Study the drawing (mm; zero at the part's minimum x, y, z) and answer. A direction names the side the tool comes from. Round coordinates to 2 decimals unless told otherwise and drop trailing zeros. Order: outer loops, then holes, each group sorted by start corner. A loop starts at its lowest first (then second) coordinate and runs counter-clockwise, first axis right, second up. Notation, with made-up numbers: (58, 4.5) - (86, 4.5) arc R17 cw to (86, 29.5) - close; hole circle Ø7 at (70, 44). An arc over 180 degrees is marked (long way). Put each result on its own line as item: value.
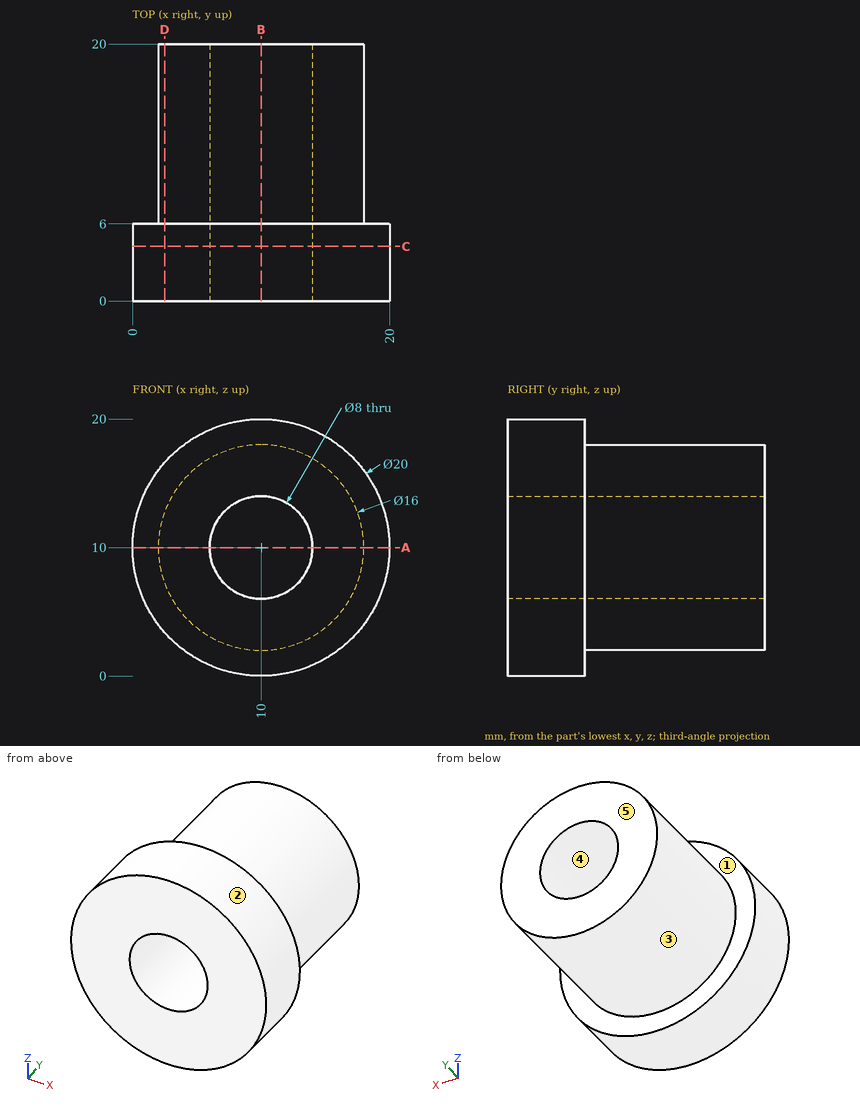
1) Straight lines are drawn through the part: L1, parallel to Z at x = 10, y = 10.25; L2, parallel to X at y = 5, z = 9.5. For each, find the intervals that lie inside material, in ascending order. Write a range as from..to.
Findings below:
L1: z = 2..6, 14..18
L2: x = 0.01..6.03, 13.97..19.99
2) A cutting plane is placed at B-B on x = 10. Write down the section's boundary in (y, z), then the cut area to 3 significant figures.
Findings below:
outline: (0, 0) - (6, 0) - (6, 2) - (20, 2) - (20, 6) - (0, 6) - close; (0, 14) - (20, 14) - (20, 18) - (6, 18) - (6, 20) - (0, 20) - close
area: 184 mm2
3) A cutting plane is placed at C-C on y = 4.25. Write down the section's boundary in (x, z).
Findings below:
outline: circle Ø20 at (10, 10); hole circle Ø8 at (10, 10)
4) Given pin 1 Ø10.5 at (x, z) = (10, 10) entering from -Y; pin 2 Ø2 at (x, y) = (16, 3.5) entering from +Z; pin 3 Ø2 at (x, y) = (5, 9) entering from +Z; pin 4 Ø1.5 at (y, z) = (4.5, 13.5) entering from +X, each flat-ended and moving along its own axis, determine where each tip first touches the part or whether it passes through.
Findings below:
pin 1: stops at y = 0
pin 2: stops at z = 18.66
pin 3: stops at z = 16.93
pin 4: stops at x = 19.61
5) A cutting plane is placed at D-D on x = 2.5. Write down the section's boundary in (y, z), then the cut area to 3 significant figures.
Findings below:
outline: (0, 3.39) - (6, 3.39) - (6, 7.22) - (20, 7.22) - (20, 12.78) - (6, 12.78) - (6, 16.61) - (0, 16.61) - close
area: 157 mm2
6) For the marked faces 1 and 2, determine the directions among +Z, -Z, +X, -X, +Y, -Y from which every point of the face is accessible in a straight line to the end or side of a thin tool.
Findings below:
face 1: +Y
face 2: +Y, -Y
7) For a pull along X with two mould halves and no side action, classify the marked faces 3, 4 and 5 as pulls with the +X half, pulls with the -X half, needs draft (parallel to the pull), parting line crosses it, or undercut.
Findings below:
face 3: parting line crosses it
face 4: undercut
face 5: needs draft
8) A cutting plane is placed at A-A on z = 10. Write down the section's boundary in (x, y), then the cut area to 3 significant figures.
Findings below:
outline: (0, 0) - (6, 0) - (6, 20) - (2, 20) - (2, 6) - (0, 6) - close; (14, 0) - (20, 0) - (20, 6) - (18, 6) - (18, 20) - (14, 20) - close
area: 184 mm2
